```python
from build123d import *
from OCP.BRepFilletAPI import BRepFilletAPI_MakeChamfer

# Parameters (mm, degrees)
SKETCH1_W           = 1219.2
SKETCH1_H           = 457.2
BOSS_EXTRUDE1_DEPTH = 11.90625
CHAMFER1_SIZE       = 368.3
CHAMFER1_SIZE2      = 558.8


with BuildPart() as part:
    # Sketch1 → Boss-Extrude1 (new body)
    with BuildSketch(Plane.XY):
        Rectangle(SKETCH1_W, SKETCH1_H)
    extrude(amount=BOSS_EXTRUDE1_DEPTH)

    # Chamfer1: one chamfer whose edges measure the first distance from different faces: ONE call of the kernel's chamfer builder (chamfer() names one face for all edges)
    chamfer1_edges_1 = [part.edges().sort_by_distance(p)[0] for p in [
        (-609.6, 228.6, 5.953125),
    ]]
    chamfer1_side_1 = [part.faces().sort_by_distance(p)[0] for p in [
        (-609.6, 0, 5.953125),
    ]]
    chamfer1_edges_2 = [part.edges().sort_by_distance(p)[0] for p in [
        (609.6, 228.6, 5.953125),
    ]]
    chamfer1_side_2 = [part.faces().sort_by_distance(p)[0] for p in [
        (609.6, 0, 5.953125),
    ]]
    chamfer1 = BRepFilletAPI_MakeChamfer(part.part.solid().wrapped)
    for e in chamfer1_edges_1:
        chamfer1.Add(CHAMFER1_SIZE, CHAMFER1_SIZE2, e.wrapped, chamfer1_side_1[0].wrapped)  # the first distance lies on this face
    for e in chamfer1_edges_2:
        chamfer1.Add(CHAMFER1_SIZE, CHAMFER1_SIZE2, e.wrapped, chamfer1_side_2[0].wrapped)  # the first distance lies on this face
    add(Compound.cast(chamfer1.Shape()), mode=Mode.REPLACE)


solid = part.part
```
Here's how the part is built. I have some questions about the finished solid (model axes, mm). Coordinates: 2 decimals unless noted, no trailing zeros. Write each loop counter-clockwise with the first axis right and the second up, starting at its lowest first coordinate (ties: lowest second). Pieces come first, ordered by that corner, then holes. Notation, with made-up numbers: (46, 81.5) -> (88, 81.5) arc R22 ccw to (88, 98.5) -> close; hole circle Ø11 at (31, -16.5). An arc over 180 degrees is marked (long way). Use a Markdown table: item, result. Add a question column.
(1) I'm going to push flat-ended pins straight in: P1, Ø4, axis at y = 179.5, z = 8.5, coming from the +X side; P2, Ø2, axis at y = -98, z = 4, coming from the -X side. Where does each tip first touch, or does it pass through?
(2) Please list where these lines run through material, in increasing order: line 1 (X direction, y = 58, z = 2.25); line 2 (Y direction, x = 483, z = 4); line 3 (Y direction, x = -380, z = 6.5).
(3) If we section it at B-B, the plane x = -379.5: Write out the boundary of the cut face in (y, z).
(4) If we section it at A-A, the plane z = 9: Write out the boundary of the cut face in (x, y).
(5) If we section it at C-C, the plane y = 101: Write out the boundary of the cut face in (x, z).
Outcome:
| question | item | result |
|---|---|---|
| 1 | P1 | stops at x = 128.33 |
| 1 | P2 | stops at x = -547.85 |
| 2 | line 1 | x = -309.64 to 309.64 |
| 2 | line 2 | y = -228.6 to -56.26 |
| 2 | line 3 | y = -228.6 to 11.63 |
| 3 | outline | (-228.6, 0) -> (11.96, 0) -> (11.96, 11.91) -> (-228.6, 11.91) -> close |
| 4 | outline | (-609.6, -228.6) -> (609.6, -228.6) -> (609.6, -139.7) -> (50.8, 228.6) -> (-50.8, 228.6) -> (-609.6, -139.7) -> close |
| 5 | outline | (-244.4, 0) -> (244.4, 0) -> (244.4, 11.91) -> (-244.4, 11.91) -> close |
